Geometry: final body of the model. Coordinates: model frame, mm. A direction names the side the tool comes from. Round coordinates to 2 decimals unless told otherwise and drop trailing zeros. Write each loop counter-clockwise with the first axis right and the second up, starting at its lowest first coordinate (ties: lowest second). Pieces come first, ordered by that corner, then holes. Notation, with made-up numbers: (-17.75, 83) -> (38.25, 83) arc R16 ccw to (38.25, 93) -> close; hole circle Ø3 at (21, -35.75). An arc over 180 degrees is marked (long way). Use one line per item in the form item = value. Start each with the question number.
1. Line query: L1, parallel to Y at x = -65.5, z = -93.5; L2, parallel to Y at x = -119, z = 60.5; L3, parallel to Z at x = -4, y = 512.5. Output: solid intervals per line, ascending.
2. Cut plane C-C, the plane z = -28.14. Return the cut outline in (x, y).
3. Pin query (flat end, axial travel): pin 1 Ø6 at (x, y) = (26, 485.5) entering from -Z; pin 2 Ø25 at (y, z) = (205.5, 113) entering from -X; pin 3 Ø4 at (x, y) = (86.5, 468.5) entering from -Z; pin 4 Ø3 at (x, z) = (-98.5, 34) entering from +Y. Return the tip coordinate at first contact, or that it passes through.
4. Cut plane D-D, the plane z = -98. Return the cut outline in (x, y), plus the area to 3 significant figures.
5. Cut plane B-B, the plane y = 49.5. Return the cut outline in (x, z).
6. Reachability of faces 1 (the face through (111, 158, -11)), 2 (the face through (-80.938, 450.917, -17.4)), 3 (the face through (75, 155, 126)), 4 (the face through (101.019, 161.918, -129.475)) from +Z, -Z, +X, -X, +Y, -Y: full face, straight path, thin tool, end or side. Return the list, or none.
```python
from build123d import *

# Parameters (mm, degrees)
CROQUIS1_W              = 260
CROQUIS1_H              = 340
SALIENTE_EXTRUIR1_DEPTH = 20
CROQUIS2_W              = 222
CROQUIS2_H              = 221
SALIENTE_EXTRUIR2_DEPTH = 280
CROQUIS3_W              = 150
CROQUIS3_H              = 86
SALIENTE_EXTRUIR3_DEPTH = 270
CHAFL_N1_SIZE           = 10
REDONDEO1_R             = 35
REDONDEO3_R             = 3


with BuildPart() as part:
    # Croquis1 → Saliente-Extruir1 (new body)
    with BuildSketch(Plane(origin=(0, 0, 0), x_dir=(1, 0, 0), z_dir=(0, 1, 0))):
        Rectangle(CROQUIS1_W, CROQUIS1_H)
    extrude(amount=SALIENTE_EXTRUIR1_DEPTH)

    # Croquis2 → Saliente-Extruir2 (add)
    with BuildSketch(Plane(origin=(0, 20, 0), x_dir=(1, 0, 0), z_dir=(0, 1, 0))):
        with Locations((0, 29.5)):
            Rectangle(CROQUIS2_W, CROQUIS2_H)
    extrude(amount=SALIENTE_EXTRUIR2_DEPTH)

    # Croquis3 → Saliente-Extruir3 (add)
    with BuildSketch(Plane(origin=(0, 20, 0), x_dir=(1, 0, 0), z_dir=(0, 1, 0))):
        with Locations((0, -124)):
            Rectangle(CROQUIS3_W, CROQUIS3_H)
    extrude(amount=SALIENTE_EXTRUIR3_DEPTH)

    # Chaflán1
    chafl_n1_edges = [part.edges().sort_by_distance(p)[0] for p in [
        (130, 10, 170),
        (-130, 10, 170),
        (-130, 10, -170),
        (130, 10, -170),
    ]]
    chamfer(chafl_n1_edges, length=CHAFL_N1_SIZE)

    # Redondeo1
    redondeo1_edges = [part.edges().sort_by_distance(p)[0] for p in [
        (-111, 160, -140),
        (111, 160, -140),
    ]]
    fillet(redondeo1_edges, radius=REDONDEO1_R)

    # Redondeo3
    redondeo3_edges = [part.edges().sort_by_distance(p)[0] for p in [
        (-93, 20, 81),
        (111, 20, -12),
        (111, 300, -12),
        (93, 20, 81),
        (-75, 20, 124),
        (-75, 155, 81),
        (75, 20, 124),
        (75, 155, 81),
        (0, 290, 81),
        (0, 20, -140),
        (0, 300, -140),
        (-111, 300, -12),
        (-100.748737342, 300, -129.748737342),
        (100.748737342, 300, -129.748737342),
        (-111, 20, -12),
        (100.748737342, 20, -129.748737342),
        (-100.748737342, 20, -129.748737342),
    ]]
    fillet(redondeo3_edges, radius=REDONDEO3_R)

    # Croquis4 → Revolución1 (revolve)
    with BuildSketch(Plane.ZY.offset(-0.86)):
        Polygon((-28.14, 300), (-130, 300), (-130, 322), (-105.64, 322), (-105.64, 384.5), (-110.64, 384.5), (-110.64, 515.5), (-105.64, 515.5), (-105.64, 608.5), (-28.14, 608.5), align=None)
    revolve(axis=Axis((0.86, 300, -28.14), (0, 1, 0)))


solid = part.part
```
Outcome:
q1.L1 = 0 to 322
q1.L2 = 0 to 20
q1.L3 = -110.5 to 54.22
q2.outline = (-130, 0) -> (130, 0) -> (130, 20) -> (114, 20) arc R3 cw to (111, 23) -> (111, 297) arc R3 ccw to (108, 300) -> (102.72, 300) -> (102.72, 322) -> (78.36, 322) -> (78.36, 384.5) -> (83.36, 384.5) -> (83.36, 515.5) -> (78.36, 515.5) -> (78.36, 608.5) -> (-76.64, 608.5) -> (-76.64, 515.5) -> (-81.64, 515.5) -> (-81.64, 384.5) -> (-76.64, 384.5) -> (-76.64, 322) -> (-101, 322) -> (-101, 300) -> (-108, 300) arc R3 ccw to (-111, 297) -> (-111, 23) arc R3 cw to (-114, 20) -> (-130, 20) -> close
q3.pin_1 = -107.61
q3.pin_2 = -75
q3.pin_3 = through
q3.pin_4 = 300
q4.outline = (-130, 0) -> (130, 0) -> (130, 20) -> (114, 20) arc R3 cw to (111, 23) -> (111, 297) arc R3 ccw to (108, 300) -> (74.99, 300) -> (74.99, 322) -> (34.41, 322) -> (34.41, 384.5) -> (44.74, 384.5) -> (44.74, 515.5) -> (34.41, 515.5) -> (34.41, 608.5) -> (-32.69, 608.5) -> (-32.69, 515.5) -> (-43.02, 515.5) -> (-43.02, 384.5) -> (-32.69, 384.5) -> (-32.69, 322) -> (-73.27, 322) -> (-73.27, 300) -> (-108, 300) arc R3 ccw to (-111, 297) -> (-111, 23) arc R3 cw to (-114, 20) -> (-130, 20) -> close
q4.area = 92,600 mm^2
q5.outline = (-111, -105) arc R35 ccw to (-76, -140) -> (76, -140) arc R35 ccw to (111, -105) -> (111, 81) -> (78, 81) arc R3 cw to (75, 84) -> (75, 167) -> (-75, 167) -> (-75, 84) arc R3 cw to (-78, 81) -> (-111, 81) -> close
q6.face_1 = +Z, -Z, +X, +Y
q6.face_2 = +Y
q6.face_3 = +Z, +X, +Y
q6.face_4 = -Z, +X, +Y
